The model under review builds one solid part; all positions refer to its coordinate system, in mm. Face numbers are marked on the shaded views. A direction names the side the tool comes from. Coordinates: 2 decimals unless noted, no trailing zeros. Write each loop counter-clockwise with the first axis right and the second up, starting at its lowest first coordinate (ties: lowest second). Pieces come first, ordered by that corner, then holes.
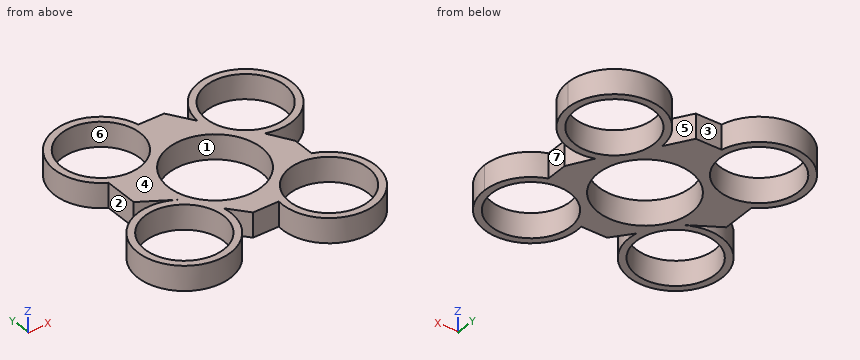
```python
from build123d import *

# Parameters (mm, degrees)
F0_R     = 11.2
F0_R_2   = 13.2
F1_DEPTH = 7


with BuildPart() as f1:
    # F0 (on Top) → F1 (new body)
    with BuildSketch(Plane.XY):
        with BuildLine():
            ThreePointArc((17.156998, 4.054863), (28.928834, 6.001855), (34.321521, 16.645437))
            ThreePointArc((34.321521, 16.645437), (21.387474, 29.842758), (7.932237, 17.177236))
            ThreePointArc((7.932237, 17.177236), (10.322797, 9.054155), (17.156998, 4.054863))
        make_face()
        with Locations((21.121521, 16.645437)):
            Circle(F0_R, mode=Mode.SUBTRACT)
        with BuildLine():
            ThreePointArc((17.156998, 4.054863), (10.322797, 9.054155), (7.932237, 17.177236))
            Line((7.932237, 17.177236), (3.535035, 24.094587))
            Line((3.535035, 24.094587), (-3.786889, 24.094587))
            ThreePointArc((-3.786889, 24.094587), (-3.533888, 22.620829), (-3.449192, 21.127913))
            ThreePointArc((-3.449192, 21.127913), (-9.966852, 9.744314), (-23.083484, 9.602294))
            Line((-23.083484, 9.602294), (-23.083484, 0))
            Line((-23.083484, 0), (-14.266823, -5.368319))
            ThreePointArc((-14.266823, -5.368319), (-10.27716, -9.131498), (-8.161303, -14.191348))
            Line((-8.161303, -14.191348), (-3.786889, -19.53627))
            Line((-3.786889, -19.53627), (3.535035, -19.53627))
            ThreePointArc((3.535035, -19.53627), (9.658903, -9.921811), (20.988215, -8.662342))
            Line((20.988215, -8.662342), (20.988215, -2.467444))
            Line((20.988215, -2.467444), (17.156998, 4.054863))
        make_face()
        Circle(F0_R_2, mode=Mode.SUBTRACT)
        with BuildLine():
            ThreePointArc((-3.449192, 21.127913), (-3.533888, 22.620829), (-3.786889, 24.094587))
            ThreePointArc((-3.786889, 24.094587), (-24.576138, 31.6827), (-23.083484, 9.602294))
            ThreePointArc((-23.083484, 9.602294), (-9.966852, 9.744314), (-3.449192, 21.127913))
        make_face()
        with Locations((-16.649192, 21.127913)):
            Circle(F0_R, mode=Mode.SUBTRACT)
        with BuildLine():
            ThreePointArc((29.839044, -21.125276), (27.401225, -13.482274), (20.988215, -8.662342))
            ThreePointArc((20.988215, -8.662342), (9.658903, -9.921811), (3.535035, -19.53627))
            ThreePointArc((3.535035, -19.53627), (15.843093, -34.301256), (29.839044, -21.125276))
        make_face()
        with Locations((16.639044, -21.125276)):
            Circle(F0_R, mode=Mode.SUBTRACT)
        with BuildLine():
            ThreePointArc((-8.161303, -14.191348), (-10.27716, -9.131498), (-14.266823, -5.368319))
            ThreePointArc((-14.266823, -5.368319), (-32.639404, -23.109021), (-7.931668, -16.6428))
            ThreePointArc((-7.931668, -16.6428), (-7.989202, -15.411708), (-8.161303, -14.191348))
        make_face()
        with Locations((-21.131668, -16.6428)):
            Circle(F0_R, mode=Mode.SUBTRACT)
    extrude(amount=F1_DEPTH)


solid = f1.part
```
Item 1: Mouldability with a two-part tool opening along X and no side actions: class the marked faces 4, 5, 6 and 7 as pulls with the +X half, pulls with the -X half, needs draft (parallel to the pull), parting line crosses it, or undercut.
Solved:
face 4: needs draft
face 5: undercut
face 6: undercut
face 7: pulls with the +X half
Item 2: Take a section at A-A, the plane x = 0. Write out the cut boundary in (y, z).
Solved:
outline: (-19.54, 0) - (-13.2, 0) - (-13.2, 7) - (-19.54, 7) - close; (13.2, 0) - (24.09, 0) - (24.09, 7) - (13.2, 7) - close
Item 3: Take a section at D-D, the plane x = 15.5. Write out the cut boundary in (y, z), plus the area to 3 significant figures.
Solved:
outline: (-34.28, 0) - (-32.27, 0) - (-32.27, 7) - (-34.28, 7) - close; (-9.98, 0) - (6.96, 0) - (6.96, 7) - (-9.98, 7) - close; (26.33, 0) - (28.59, 0) - (28.59, 7) - (26.33, 7) - close
area: 148 mm2
Item 4: For pin 1 (1 mm diameter, centred on x = 6.5, z = 4, fed in from +Y); pin 2 (4 mm diameter, centred on x = 1.5, z = 1, fed in from +Y); pin 3 (3.5 mm diameter, centred on y = 5, z = 3.5, fed in from -X), all flat-tipped, find the tip position at first contact; note any pin that passes through.
Solved:
pin 1: stops at y = 20.22
pin 2: stops at y = 24.09
pin 3: stops at x = -23.08
Item 5: To check wall thickness, follow line 1 along Y through (x, z) = (0, 3.25); line 2 along X through (y, z) = (-20.5, 5); line 3 along X through (y, z) = (-24, 2.75). State the ranges of each line that lie inside material, in increasing order.
Solved:
line 1: y = -19.54 to -13.2, 13.2 to 24.09
line 2: x = -33.76 to -31.65, -10.62 to -8.51, 3.45 to 5.46, 27.82 to 29.82
line 3: x = -32.09 to -29.58, -12.69 to -10.17, 3.76 to 5.81, 27.46 to 29.52
Item 6: Take a section at C-C, the plane x = -16.5. Write out the cut boundary in (y, z), plus the area to 3 significant figures.
Solved:
outline: (-29, 0) - (-26.84, 0) - (-26.84, 7) - (-29, 7) - close; (-6.45, 0) - (-4.28, 0) - (-4.28, 7) - (-6.45, 7) - close; (-4.01, 0) - (9.93, 0) - (9.93, 7) - (-4.01, 7) - close; (32.33, 0) - (34.33, 0) - (34.33, 7) - (32.33, 7) - close
area: 142 mm2
Item 7: Take a section at B-B, the plane y = -22.5. Write out the cut boundary in (x, z).
Solved:
outline: (-32.96, 0) - (-30.68, 0) - (-30.68, 7) - (-32.96, 7) - close; (-11.59, 0) - (-9.3, 0) - (-9.3, 7) - (-11.59, 7) - close; (3.51, 0) - (5.52, 0) - (5.52, 7) - (3.51, 7) - close; (27.75, 0) - (29.77, 0) - (29.77, 7) - (27.75, 7) - close
Item 8: Machinability: for the marked faces 1, 2 and 3, which of the approach directions +Z, -Z, +X, -X, +Y, -Y give a long, thin tool a straight path to every point of the face, cutting with its end or side? Answer none if there is none.
Solved:
face 1: +Z, -Z
face 2: +Z, -Z, -X
face 3: +Z, -Z, +Y
